Design review of the part built by this model. Coordinates are the model's own, in mm. Face numbers are marked on the shaded views. A direction names the side the tool comes from. Give positions to 0.01 mm unless a question says otherwise; leave off trailing zeros. Write each loop counter-clockwise with the first axis right and the second up, starting at its lowest first coordinate (ties: lowest second). Pieces come first, ordered by that corner, then holes. Notation, with made-up numbers: (-7.5, 44) - (45.5, 44) arc R12 cw to (45.5, 55) - close; hole circle Ø11 at (64, -6.5). An arc over 180 degrees is marked (long way). Use a Markdown table: item, result. Add a question column.
Autodesk Inventor part; units mm, degrees
ref_plane "YZ Plane" through (0, 0, 0) normal (1, 0, 0) x (0, 1, 0)
ref_plane "XZ Plane" through (0, 0, 0) normal (0, 1, 0) x (-1, 0, 0)
ref_plane "XY Plane" through (0, 0, 0) normal (0, 0, 1) x (1, 0, 0)
sketch "Sketch1" plane through (0, 0, 0) normal (0, 0, 1) x (1, 0, 0)
  circle A0 centre (0, 0) radius 11
  line L0 (-7.7, 0) -> (7.7, 0) construction
  circle A1 centre (-7.7, 0) radius 1.25
  circle A2 centre (7.7, 0) radius 1.25
  dimension "d0" = 22
  dimension "d1" = 15.4
  dimension "d2" = 2.5
  dimension "d3" = 2.5
extrude "Extrusion1" add sketch "Sketch1" along normal blind 3
sketch "Sketch2" plane through (0, 0, 3) normal (0, 0, 1) x (1, 0, 0)
  circle A0 centre (0, 0) radius 11
  arc A1 (6.6742, -8.8894) -> (0, -4) centre (0, -11) ccw
  arc A2 (0, -4) -> (-6.6426, -8.7919) centre (0, -11) ccw
  point P0 (-6.6362, -8.7727)
  point P1 (6.6362, -8.7727)
extrude "Extrusion2" cut sketch "Sketch2" against normal blind 10 contours A2 A1 A0 picked at (-1.3613, -8.6538)
equation "\"d0\" = cs_diam"
equation "\"d1\" = cs_holeSpacing"
equation "\"d2\" = cs_holeDiam"
equation "\"d3\" = cs_holeDiam"
equation "\"d4\" = cs_depth"
equation "\"cs_diam\" = 22"
equation "\"cs_holeSpacing\" = 15.4"
equation "\"cs_holeDiam\" = 2.5"
equation "\"cs_depth\" = 3"
properties part number "Caster Spacer 3mm" material "PMMA Plastic"
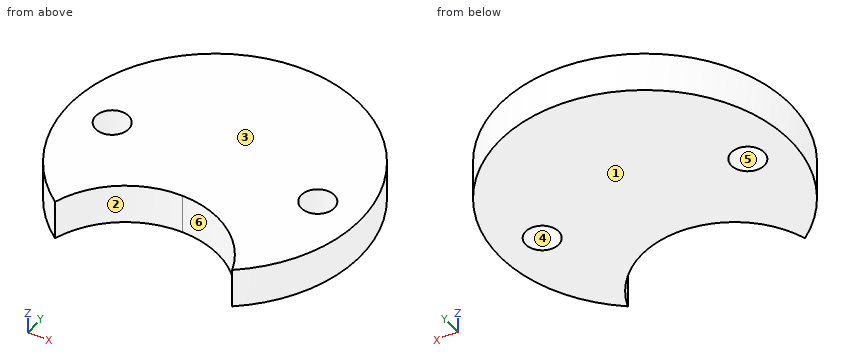
(1) Tool access review of the marked faces 1 and 2: name each direction out of +Z, -Z, +X, -X, +Y, -Y from which nothing blocks a thin tool from reaching the whole face with its end or side.
(2) Add section D-D (y = 0). State the section outline as (x, z) points.
(3) Add section C-C (z = 1.35). State the section outline as (x, y) points.
(4) Add section B-B (y = -5.5). State the section outline as (x, z) points.
(5) Mouldability with a two-part tool opening along Y and no side actions: class the marked faces 3, 4, 5 and 6 as +Y half, -Y half, draft (parallel to the pull), parting line (faces both ways), or undercut.
(6) Insertion check: pin 1 (2 mm diameter, centred on x = -7.7, y = 0, fed in from +Z); pin 2 (1.5 mm diameter, centred on x = 4.5, z = 1.5, fed in from -Y). Each pin has a flat end and moves straight along its axis. Give the tip position at first contact, or say it passes through.
(7) Add section A-A (x = -7.7). State the section outline as (y, z) points, and give its area (3 significant figures).
(8) For line 1 along Y through (x, z) = (-7.7, 1.8); line 2 along Y through (x, z) = (7, 1.2); line 3 along Y through (x, z) = (9.75, 1.7), list the stretches that pass through material, from the lowest coordinate up.
Answers follow:
| question | item | result |
|---|---|---|
| 1 | face 1 | -Z, +X, -X, +Y, -Y |
| 1 | face 2 | +Z, -Z, -Y |
| 2 | outline | (-11, 0) - (-8.95, 0) - (-8.95, 3) - (-11, 3) - close; (-6.45, 0) - (6.45, 0) - (6.45, 3) - (-6.45, 3) - close; (8.95, 0) - (11, 0) - (11, 3) - (8.95, 3) - close |
| 3 | outline | (-6.64, -8.77) arc R7 cw to (0, -4) arc R7 cw to (6.64, -8.77) arc R11 ccw (long way) to start; hole circle Ø2.5 at (-7.7, 0); hole circle Ø2.5 at (7.7, 0) |
| 4 | outline | (-9.53, 0) - (-4.33, 0) - (-4.33, 3) - (-9.53, 3) - close; (4.33, 0) - (9.53, 0) - (9.53, 3) - (4.33, 3) - close |
| 5 | face 3 | draft |
| 5 | face 4 | undercut |
| 5 | face 5 | undercut |
| 5 | face 6 | -Y half |
| 6 | pin 1 | through |
| 6 | pin 2 | y = -6.37 |
| 7 | outline | (-7.86, 0) - (-1.25, 0) - (-1.25, 3) - (-7.86, 3) - close; (1.25, 0) - (7.86, 0) - (7.86, 3) - (1.25, 3) - close |
| 7 | area | 39.6 mm^2 |
| 8 | line 1 | -7.86 to -1.25, 1.25 to 7.86 |
| 8 | line 2 | -8.49 to -1.04, 1.04 to 8.49 |
| 8 | line 3 | -5.09 to 5.09 |
